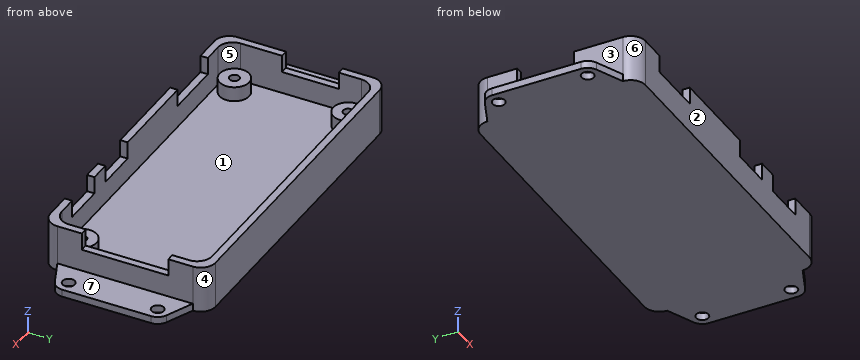
```python
from build123d import *

# Parameters (mm, degrees)
F0_R     = 3
F0_W     = 19
F0_H     = 1.5
F0_R_2   = 1
F0_W_2   = 1.5
F0_H_2   = 17.5
F0_H_3   = 11.5
F0_W_3   = 11.5
F0_W_4   = 8.5
F0_W_5   = 4.1
F1_DEPTH = 1.5
F2_DEPTH = 3
F3_DEPTH = 8
F4_DEPTH = 4.5
F5_R     = 1.25
F6_DEPTH = 1.5


with BuildPart() as f1:
    # F0 (on Top) → F1 (new body)
    with BuildSketch(Plane.XY):
        with BuildLine():
            Line((29.7, 15.2), (-29.7, 15.2))
            ThreePointArc((-29.7, 15.2), (-31.8213203436, 14.3213203436), (-32.7, 12.2))
            Line((-32.7, 12.2), (-32.7, 7.65))
            Line((-32.7, 7.65), (-32.7, -3.85))
            Line((-32.7, -3.85), (-32.7, -12.2))
            ThreePointArc((-32.7, -12.2), (-31.8213203436, -14.3213203436), (-29.7, -15.2))
            Line((-29.7, -15.2), (-25.85, -15.2))
            Line((-25.85, -15.2), (-14.35, -15.2))
            Line((-14.35, -15.2), (4.65, -15.2))
            Line((4.65, -15.2), (13.15, -15.2))
            Line((13.15, -15.2), (17.25, -15.2))
            Line((17.25, -15.2), (25.75, -15.2))
            Line((25.75, -15.2), (29.7, -15.2))
            ThreePointArc((29.7, -15.2), (31.8213203436, -14.3213203436), (32.7, -12.2))
            Line((32.7, -12.2), (32.7, -8.75))
            Line((32.7, -8.75), (32.7, 8.75))
            Line((32.7, 8.75), (32.7, 12.2))
            ThreePointArc((32.7, 12.2), (31.8213203436, 14.3213203436), (29.7, 15.2))
        make_face()
        with Locations((-29, -11.5)):
            Circle(F0_R, mode=Mode.SUBTRACT)
        with Locations((29, -11.5)):
            Circle(F0_R, mode=Mode.SUBTRACT)
        with Locations((-29, 11.5)):
            Circle(F0_R, mode=Mode.SUBTRACT)
        with Locations((29, 11.5)):
            Circle(F0_R, mode=Mode.SUBTRACT)
        with BuildLine():
            ThreePointArc((-32.7, 12.2), (-31.8213203436, 14.3213203436), (-29.7, 15.2))
            Line((-29.7, 15.2), (29.7, 15.2))
            ThreePointArc((29.7, 15.2), (31.8213203436, 14.3213203436), (32.7, 12.2))
            Line((32.7, 12.2), (32.7, 8.75))
            Line((32.7, 8.75), (34.2, 8.75))
            Line((34.2, 8.75), (34.2, 13.7))
            ThreePointArc((34.2, 13.7), (33.3213203436, 15.8213203436), (31.2, 16.7))
            Line((31.2, 16.7), (-31.2, 16.7))
            ThreePointArc((-31.2, 16.7), (-33.3213203436, 15.8213203436), (-34.2, 13.7))
            Line((-34.2, 13.7), (-34.2, 7.65))
            Line((-34.2, 7.65), (-32.7, 7.65))
            Line((-32.7, 7.65), (-32.7, 12.2))
        make_face()
        with BuildLine():
            Line((-32.7, -12.2), (-32.7, -3.85))
            Line((-32.7, -3.85), (-34.2, -3.85))
            Line((-34.2, -3.85), (-34.2, -13.7))
            ThreePointArc((-34.2, -13.7), (-33.3213203436, -15.8213203436), (-31.2, -16.7))
            Line((-31.2, -16.7), (-25.85, -16.7))
            Line((-25.85, -16.7), (-25.85, -15.2))
            Line((-25.85, -15.2), (-29.7, -15.2))
            ThreePointArc((-29.7, -15.2), (-31.8213203436, -14.3213203436), (-32.7, -12.2))
        make_face()
        with Locations((-4.85, -15.95)):
            Rectangle(F0_W, F0_H)
        with Locations((-29, -11.5)):
            Circle(F0_R)
        with Locations((-29, -11.5)):
            Circle(F0_R_2, mode=Mode.SUBTRACT)
        with Locations((-29, 11.5)):
            Circle(F0_R)
        with Locations((-29, 11.5)):
            Circle(F0_R_2, mode=Mode.SUBTRACT)
        with Locations((29, -11.5)):
            Circle(F0_R)
        with Locations((29, -11.5)):
            Circle(F0_R_2, mode=Mode.SUBTRACT)
        with Locations((29, 11.5)):
            Circle(F0_R)
        with Locations((29, 11.5)):
            Circle(F0_R_2, mode=Mode.SUBTRACT)
        with Locations((33.45, 0)):
            Rectangle(F0_W_2, F0_H_2)
        with BuildLine():
            Line((34.2, -8.75), (32.7, -8.75))
            Line((32.7, -8.75), (32.7, -12.2))
            ThreePointArc((32.7, -12.2), (31.8213203436, -14.3213203436), (29.7, -15.2))
            Line((29.7, -15.2), (25.75, -15.2))
            Line((25.75, -15.2), (25.75, -16.7))
            Line((25.75, -16.7), (31.2, -16.7))
            ThreePointArc((31.2, -16.7), (33.3213203436, -15.8213203436), (34.2, -13.7))
            Line((34.2, -13.7), (34.2, -8.75))
        make_face()
        with Locations((-33.45, 1.9)):
            Rectangle(F0_W_2, F0_H_3)
        with Locations((-20.1, -15.95)):
            Rectangle(F0_W_3, F0_H)
        with Locations((21.5, -15.95)):
            Rectangle(F0_W_4, F0_H)
        with Locations((8.9, -15.95)):
            Rectangle(F0_W_4, F0_H)
        with Locations((15.2, -15.95)):
            Rectangle(F0_W_5, F0_H)
        with Locations((-29, -11.5)):
            Circle(F0_R_2)
        with Locations((-29, 11.5)):
            Circle(F0_R_2)
        with Locations((29, -11.5)):
            Circle(F0_R_2)
        with Locations((29, 11.5)):
            Circle(F0_R_2)
    extrude(amount=-F1_DEPTH)

    # F0 (on Top) → F2 (join)
    with BuildSketch(Plane.XY):
        with Locations((-29, 11.5)):
            Circle(F0_R)
        with Locations((-29, 11.5)):
            Circle(F0_R_2, mode=Mode.SUBTRACT)
        with Locations((-29, -11.5)):
            Circle(F0_R)
        with Locations((-29, -11.5)):
            Circle(F0_R_2, mode=Mode.SUBTRACT)
        with Locations((29, 11.5)):
            Circle(F0_R)
        with Locations((29, 11.5)):
            Circle(F0_R_2, mode=Mode.SUBTRACT)
        with Locations((29, -11.5)):
            Circle(F0_R)
        with Locations((29, -11.5)):
            Circle(F0_R_2, mode=Mode.SUBTRACT)
    extrude(amount=F2_DEPTH)

    # F0 (on Top) → F3 (join)
    with BuildSketch(Plane.XY):
        with BuildLine():
            Line((-32.7, -12.2), (-32.7, -3.85))
            Line((-32.7, -3.85), (-34.2, -3.85))
            Line((-34.2, -3.85), (-34.2, -13.7))
            ThreePointArc((-34.2, -13.7), (-33.3213203436, -15.8213203436), (-31.2, -16.7))
            Line((-31.2, -16.7), (-25.85, -16.7))
            Line((-25.85, -16.7), (-25.85, -15.2))
            Line((-25.85, -15.2), (-29.7, -15.2))
            ThreePointArc((-29.7, -15.2), (-31.8213203436, -14.3213203436), (-32.7, -12.2))
        make_face()
        with BuildLine():
            ThreePointArc((-32.7, 12.2), (-31.8213203436, 14.3213203436), (-29.7, 15.2))
            Line((-29.7, 15.2), (29.7, 15.2))
            ThreePointArc((29.7, 15.2), (31.8213203436, 14.3213203436), (32.7, 12.2))
            Line((32.7, 12.2), (32.7, 8.75))
            Line((32.7, 8.75), (34.2, 8.75))
            Line((34.2, 8.75), (34.2, 13.7))
            ThreePointArc((34.2, 13.7), (33.3213203436, 15.8213203436), (31.2, 16.7))
            Line((31.2, 16.7), (-31.2, 16.7))
            ThreePointArc((-31.2, 16.7), (-33.3213203436, 15.8213203436), (-34.2, 13.7))
            Line((-34.2, 13.7), (-34.2, 7.65))
            Line((-34.2, 7.65), (-32.7, 7.65))
            Line((-32.7, 7.65), (-32.7, 12.2))
        make_face()
        with Locations((-4.85, -15.95)):
            Rectangle(F0_W, F0_H)
        with Locations((15.2, -15.95)):
            Rectangle(F0_W_5, F0_H)
        with BuildLine():
            Line((34.2, -8.75), (32.7, -8.75))
            Line((32.7, -8.75), (32.7, -12.2))
            ThreePointArc((32.7, -12.2), (31.8213203436, -14.3213203436), (29.7, -15.2))
            Line((29.7, -15.2), (25.75, -15.2))
            Line((25.75, -15.2), (25.75, -16.7))
            Line((25.75, -16.7), (31.2, -16.7))
            ThreePointArc((31.2, -16.7), (33.3213203436, -15.8213203436), (34.2, -13.7))
            Line((34.2, -13.7), (34.2, -8.75))
        make_face()
    extrude(amount=F3_DEPTH)

    # F0 (on Top) → F4 (join)
    with BuildSketch(Plane.XY):
        with Locations((-33.45, 1.9)):
            Rectangle(F0_W_2, F0_H_3)
        with Locations((-20.1, -15.95)):
            Rectangle(F0_W_3, F0_H)
        with Locations((8.9, -15.95)):
            Rectangle(F0_W_4, F0_H)
        with Locations((21.5, -15.95)):
            Rectangle(F0_W_4, F0_H)
        with Locations((33.45, 0)):
            Rectangle(F0_W_2, F0_H_2)
    extrude(amount=F4_DEPTH)

    # F5 (on face) → F6 (join)
    with BuildSketch(Plane.XY):
        with BuildLine():
            Line((39.7029067074, 11.2900170603), (34.2, 13.7))
            Line((34.2, 13.7), (34.2, -13.7))
            Line((34.2, -13.7), (39.7029067074, -11.2900170603))
            ThreePointArc((39.7029067074, -11.2900170603), (36.607481569, -7.6320209739), (41.2, -9))
            Line((41.2, -9), (41.2, 9))
            ThreePointArc((41.2, 9), (36.607481569, 7.6320209739), (39.7029067074, 11.2900170603))
        make_face()
        with BuildLine():
            ThreePointArc((41.2, -9), (36.607481569, -7.6320209739), (39.7029067074, -11.2900170603))
            ThreePointArc((39.7029067074, -11.2900170603), (40.792518431, -10.3679790261), (41.2, -9))
        make_face()
        with Locations((38.7, -9)):
            Circle(F5_R, mode=Mode.SUBTRACT)
        with BuildLine():
            ThreePointArc((41.2, 9), (40.792518431, 10.3679790261), (39.7029067074, 11.2900170603))
            ThreePointArc((39.7029067074, 11.2900170603), (36.607481569, 7.6320209739), (41.2, 9))
        make_face()
        with Locations((38.7, 9)):
            Circle(F5_R, mode=Mode.SUBTRACT)
        with BuildLine():
            Line((-34.2, -13.7), (-34.2, 13.7))
            Line((-34.2, 13.7), (-39.7029067074, 11.2900170603))
            ThreePointArc((-39.7029067074, 11.2900170603), (-37.3320209739, 11.092518431), (-36.2, 9))
            ThreePointArc((-36.2, 9), (-38.7, 6.5), (-41.2, 9))
            Line((-41.2, 9), (-41.2, -9))
            ThreePointArc((-41.2, -9), (-38.7, -6.5), (-36.2, -9))
            ThreePointArc((-36.2, -9), (-37.3320209739, -11.092518431), (-39.7029067074, -11.2900170603))
            Line((-39.7029067074, -11.2900170603), (-34.2, -13.7))
        make_face()
        with BuildLine():
            ThreePointArc((-36.2, 9), (-37.3320209739, 11.092518431), (-39.7029067074, 11.2900170603))
            ThreePointArc((-39.7029067074, 11.2900170603), (-40.792518431, 10.3679790261), (-41.2, 9))
            ThreePointArc((-41.2, 9), (-38.7, 6.5), (-36.2, 9))
        make_face()
        with Locations((-38.7, 9)):
            Circle(F5_R, mode=Mode.SUBTRACT)
        with BuildLine():
            ThreePointArc((-41.2, -9), (-40.792518431, -10.3679790261), (-39.7029067074, -11.2900170603))
            ThreePointArc((-39.7029067074, -11.2900170603), (-37.3320209739, -11.092518431), (-36.2, -9))
            ThreePointArc((-36.2, -9), (-38.7, -6.5), (-41.2, -9))
        make_face()
        with Locations((-38.7, -9)):
            Circle(F5_R, mode=Mode.SUBTRACT)
    extrude(amount=-F6_DEPTH)


solid = f1.part
```
Source: CAD feature listing. Evaluate the final solid. Frame: model axes, mm. Face numbers are marked on the shaded views. A direction names the side the tool comes from. Round coordinates to 2 decimals unless told otherwise and drop trailing zeros. Loops run counter-clockwise (first coordinate to the right, second up) from the corner with the lowest first, then second, coordinate; pieces in that order, holes last. Notation, with made-up numbers: M 16.25,-37.5 L 32.25,-37.5 A25 ccw 32.25,-6.5 Z; hole C 50.25,18 d9. An arc over 180 degrees is marked long. Use a Markdown table: item, result. Add a question column.
1. Contact query for flat-ended pins moving along their axis: pin 1 (12 mm diameter, centred on x = 32, y = -7, fed in from +Z); pin 2 (1.8 mm diameter, centred on x = -30.5, y = 13, fed in from +Z); pin 3 (0.8 mm diameter, centred on x = 33.5, z = 5.5, fed in from +Y); pin 4 (2 mm diameter, centred on x = 36.5, y = -6.5, fed in from +Z). Output: stop coordinate, or through.
2. Set-up query: the marked faces 5, 6 and 7. Return all of +Z, -Z, +X, -X, +Y, -Y with unobstructed straight access to the full face (end or side cutting, diameter ignored); none if empty.
3. Ray query, line 1 along Y through (x, z) = (29, 0.6); line 2 along X through (y, z) = (10.5, 5); line 3 along Y through (x, z) = (25.5, 3). Return the intervals inside material, ascending. Write a range as [from, to].
4. Pull-direction query (X, two-part tool) for the marked faces 1, 2, 3 and 4; classes: +X half, -X half, draft (parallel to the pull), parting line (faces both ways), or undercut.
5. Cut plane B-B, the plane y = 0.5. Output: boundary loops of the cut face in (x, z), and give its area (3 significant figures).
6. Cut plane C-C, the plane x = -38.7. Output: boundary loops of the cut face in (y, z), and give its area (3 significant figures).
7. Cut plane A-A, the plane z = 1. State how many separate pieces and enclosed holes the cut face has, and give its area (3 significant figures).
8. Cut plane D-D, the plane x = -20.5. Output: boundary loops of the cut face in (y, z), and give its area (4 significant figures).
Solution:
| question | item | result |
|---|---|---|
| 1 | pin 1 | stops at z = 8 |
| 1 | pin 2 | stops at z = 3 |
| 1 | pin 3 | stops at y = 16.02 |
| 1 | pin 4 | stops at z = 0 |
| 2 | face 5 | +Z |
| 2 | face 6 | +Z, -Z, -X, -Y |
| 2 | face 7 | +Z, +X, +Y, -Y |
| 3 | line 1 | y = [-16.7, -15.2], [-14.5, -12.5], [-10.5, -8.5], [8.5, 10.5], [12.5, 14.5], [15.2, 16.7] |
| 3 | line 2 | x = [-34.2, -32.7], [32.7, 34.2] |
| 3 | line 3 | y = [-16.7, -15.2], [15.2, 16.7] |
| 4 | face 1 | undercut |
| 4 | face 2 | draft |
| 4 | face 3 | -X half |
| 4 | face 4 | +X half |
| 5 | outline | M -41.2,-1.5 L 41.2,-1.5 L 41.2,0 L 34.2,0 L 34.2,4.5 L 32.7,4.5 L 32.7,0 L -32.7,0 L -32.7,4.5 L -34.2,4.5 L -34.2,0 L -41.2,0 Z |
| 5 | area | 137 mm2 |
| 6 | outline | M -11.73,-1.5 L -10.25,-1.5 L -10.25,0 L -11.73,0 Z; M -7.75,-1.5 L 7.75,-1.5 L 7.75,0 L -7.75,0 Z; M 10.25,-1.5 L 11.73,-1.5 L 11.73,0 L 10.25,0 Z |
| 6 | area | 27.7 mm2 |
| 7 | separate pieces | 5 |
| 7 | enclosed holes | 5 |
| 7 | area | 397 mm2 |
| 8 | outline | M -16.7,-1.5 L 16.7,-1.5 L 16.7,8 L 15.2,8 L 15.2,0 L -15.2,0 L -15.2,4.5 L -16.7,4.5 Z |
| 8 | area | 68.85 mm2 |
